```python
from build123d import *

# Parameters (mm, degrees)
BOSS_EXTRUDE1_DEPTH = 2.38125
FILLET1_R           = 2.54
FILLET2_R           = 2.54
SKETCH2_R           = 4.7625
BOSS_EXTRUDE2_DEPTH = 3.96875
FILLET3_R           = 0.635
SKETCH3_R           = 3.175
CUT_EXTRUDE1_DEPTH  = 6.35
SKETCH4_R           = 0.79375
CUT_EXTRUDE2_DEPTH  = 6.35


with BuildPart() as part:
    # Sketch1 → Boss-Extrude1 (new body)
    with BuildSketch(Plane(origin=(0, 0, 0), x_dir=(1, 0, 0), z_dir=(0, 1, 0))):
        with BuildLine():
            Line((4.089179599, 4.858097386), (16.271875, 2.778125))
            ThreePointArc((16.271875, 2.778125), (19.05, 0), (16.271875, -2.778125))
            Line((16.271875, -2.778125), (4.089179599, -4.858097386))
            ThreePointArc((4.089179599, -4.858097386), (0, -6.35), (-4.089179599, -4.858097386))
            Line((-4.089179599, -4.858097386), (-16.271875, -2.778125))
            ThreePointArc((-16.271875, -2.778125), (-19.05, 0), (-16.271875, 2.778125))
            Line((-16.271875, 2.778125), (-4.089179599, 4.858097386))
            ThreePointArc((-4.089179599, 4.858097386), (0, 6.35), (4.089179599, 4.858097386))
        make_face()
    extrude(amount=BOSS_EXTRUDE1_DEPTH)

    # Fillet1
    fillet1_edges = [part.edges().sort_by_distance(p)[0] for p in [
        (16.271875, 1.190625, -2.778125),
        (16.271875, 1.190625, 2.778125),
        (-16.271875, 1.190625, 2.778125),
        (-16.271875, 1.190625, -2.778125),
    ]]
    fillet(fillet1_edges, radius=FILLET1_R)

    # Fillet2
    fillet2_edges = [part.edges().sort_by_distance(p)[0] for p in [
        (4.089179599, 1.190625, -4.858097386),
        (4.089179599, 1.190625, 4.858097386),
        (-4.089179599, 1.190625, 4.858097386),
        (-4.089179599, 1.190625, -4.858097386),
    ]]
    fillet(fillet2_edges, radius=FILLET2_R)

    # Sketch2 → Boss-Extrude2 (add)
    with BuildSketch(Plane(origin=(0, 2.38125, 0), x_dir=(1, 0, 0), z_dir=(0, 1, 0))):
        with Locations(Location((0, 0, 0), (0, 0, 270))):
            Circle(SKETCH2_R)
    extrude(amount=BOSS_EXTRUDE2_DEPTH)

    # Fillet3
    fillet3_edges = [part.edges().sort_by_distance(p)[0] for p in [
        (0, 2.38125, -4.7625),
    ]]
    fillet(fillet3_edges, radius=FILLET3_R)

    # Sketch3 → Cut-Extrude1 (cut)
    with BuildSketch(Plane(origin=(0, 6.35, 0), x_dir=(1, 0, 0), z_dir=(0, 1, 0))):
        with Locations(Location((0, 0, 0), (0, 0, 270))):
            Circle(SKETCH3_R)
    extrude(amount=-CUT_EXTRUDE1_DEPTH, mode=Mode.SUBTRACT)

    # Sketch4 → Cut-Extrude2 (cut)
    with BuildSketch(Plane(origin=(0, 2.38125, 0), x_dir=(1, 0, 0), z_dir=(0, 1, 0))):
        with Locations(Location((9.525, 0, 0), (0, 0, 270))):
            Circle(SKETCH4_R)
        with Locations(Location((-9.525, 0, 0), (0, 0, 270))):
            Circle(SKETCH4_R)
        with Locations(Location((12.7, 0, 0), (0, 0, 270))):
            Circle(SKETCH4_R)
        with Locations(Location((15.875, 0, 0), (0, 0, 270))):
            Circle(SKETCH4_R)
        with Locations(Location((-12.7, 0, 0), (0, 0, 270))):
            Circle(SKETCH4_R)
        with Locations(Location((-15.875, 0, 0), (0, 0, 270))):
            Circle(SKETCH4_R)
    extrude(amount=-CUT_EXTRUDE2_DEPTH, mode=Mode.SUBTRACT)


solid = part.part
```
Check sheet for the modelled part. Datum: model origin and axes. Units: mm. A direction names the side the tool comes from. Round coordinates to 2 decimals unless told otherwise and drop trailing zeros. Loops run counter-clockwise (first coordinate to the right, second up) from the corner with the lowest first, then second, coordinate; pieces in that order, holes last. Notation, with made-up numbers: (-29.5, 62) - (14.5, 62) arc R22 ccw to (14.5, 100) - close; hole circle Ø2 at (13, -33). An arc over 180 degrees is marked (long way). Write item = value, one per line. Start each with the question number.
Q1. Section check D-D (x = -12.7). Record the boundary of the cut face in (y, z), plus the area to 3 significant figures.
Q2. Thickness scan on L1, parallel to X at y = 5, z = 0 (1 decimal); L2, parallel to X at y = 4.75, z = 1.25; L3, parallel to Z at x = -1, y = 5. Record the ranges inside material, lowest first.
Q3. Section check C-C (z = 0). Count the separate pieces of the cut face and the enclosed holes in it, plus the area to 3 significant figures.
Q4. Release check for a two-part mould opening along X. For faces 3 (the face through (-8.86, 1.21, 0.43)), 4 (the face through (-4, 0, 0)), 5 (the face through (10.322, 1.174, -3.794)), 6 (the face through (-0.05, 1.17, -6.35)) record: pulls with the +X half, pulls with the -X half, needs draft (parallel to the pull), parting line crosses it, or undercut.
Q5. Access from +Z, -Z, +X, -X, +Y, -Y to the whole of each face (thin tool, end or side, straight path). Record for faces 1 (the face through (-11.913, 1.207, -0.103)), 2 (the face through (-2.9, 4.66, -3.78)).
Q6. Depth check by flat-ended pin: P1, Ø1, axis at x = -15.875, z = 0, coming from the -Y side; P2, Ø3, axis at x = 13, z = -3.5, coming from the +Y side; P3, Ø3, axis at y = 3, z = -3, coming from the +X side; P4, Ø1, axis at y = 3.5, z = -1, coming from the -X side. Enter the tip coordinate at first touch or a pass-through.
Derived:
q1.outline = (0, -3.39) - (2.38, -3.39) - (2.38, -0.79) - (0, -0.79) - close; (0, 0.79) - (2.38, 0.79) - (2.38, 3.39) - (0, 3.39) - close
q1.area = 12.4 mm^2
q2.L1 = -4.8 to -3.2, 3.2 to 4.8
q2.L2 = -4.6 to -2.92, 2.92 to 4.6
q2.L3 = -4.66 to -3.01, 3.01 to 4.66
q3.separate_pieces = 8
q3.enclosed_holes = 0
q3.area = 65.7 mm^2
q4.face_3 = undercut
q4.face_4 = needs draft
q4.face_5 = pulls with the +X half
q4.face_6 = parting line crosses it
q5.face_1 = +Y, -Y
q5.face_2 = +Y
q6.P1 = through
q6.P2 = 2.38
q6.P3 = 18.52
q6.P4 = -4.74
